Could you check a few things on this model? Use its own coordinates, in mm. A direction names the side the tool comes from. Coordinates: 2 decimals unless noted, no trailing zeros. Order: outer loops, then holes, each group sorted by start corner. A loop starts at its lowest first (then second) coordinate and runs counter-clockwise, first axis right, second up. Notation, with made-up numbers: (-25, -28.5) -> (-2, -28.5) arc R27 cw to (-2, 6.5) -> close; hole circle Ø4 at (9.25, -11.75). An arc over 180 degrees is marked (long way). Put each result on its own line as item: value. Start each with the question number.
Q1. Please list where these lines run through material, in increasing order: line 1 along X through (y, z) = (6, -63); line 2 along X through (y, z) = (5.4, 63.5); line 3 along Z through (x, y) = (111.5, 19.5).
Q2. Will these pins go through, and if not, where does the flat tip stop? pin 1 (19.5 mm diameter, centred on x = 145, y = 20.5, fed in from +Z); pin 2 (11 mm diameter, centred on x = 207.5, z = -66.5, fed in from +Y); pin 3 (4 mm diameter, centred on x = 31.5, z = 49, fed in from +Y).
Q3. For faces 1 (the face through (150, 4.382, 65)), 2 (the face through (150, 38.227, -1)), which set-ups out of +Z, -Z, +X, -X, +Y, -Y let a thin tool reach every point of the face, with its end or its side?
Q4. If we section it at D-D (z = -39): Please give me the cut outline in (x, y) (3 decimals), and give its area (3 significant figures).
Q5. If we section it at A-A (y = 30.5): Please give me the cut outline in (x, z), and give its area (3 significant figures).
Q6. If we section it at C-C (z = 20.5): Please give me the cut outline in (x, y) (3 decimals), and give its area (3 significant figures).
Q7. We'd pull the mould along Z, two halves only. Please class faces 3 (the face through (150.27, 6.25, 49.53)), 4 (the face through (150, 7.43, -65)), 5 (the face through (150, 23, -50.8)): +Z half, -Z half, draft (parallel to the pull), parting line (faces both ways), or undercut.
from build123d import *

# Parameters (mm, degrees)
BOSS_EXTRUDE1_DEPTH              = 304.8
SKETCH2_R                        = 2.3876
CUT_EXTRUDE1_DEPTH               = 317.354227758
SKETCH3_R                        = 9.525
CUT_EXTRUDE2_DEPTH               = 304.8
LPATTERN1_COUNT                  = 2
LPATTERN1_PITCH                  = 171.958
FILLET1_R                        = 6.35
CONVERT_SOLID1_DEPTH             = 304.8
F_10_0_1935_DIAMETER_HOLE1_D     = 4.9149
F_10_0_1935_DIAMETER_HOLE1_DEPTH = 3.048


# Read off the part's stored shape, not the designer's step: Convert-Solid1
with BuildPart() as part:
    # Sketch1 → Boss-Extrude1 (new body)
    with BuildSketch(Plane(origin=(0, 0, 0), x_dir=(0, 0, -1), z_dir=(1, 0, 0))):
        with BuildLine():
            Line((-76.2, 4.2545), (-53.975, 4.2545))
            ThreePointArc((-53.975, 4.2545), (-49.484871939, 6.114371939), (-47.625, 10.6045))
            Line((-47.625, 10.6045), (-47.625, 34.925))
            ThreePointArc((-47.625, 34.925), (-46.69506403, 37.17006403), (-44.45, 38.1))
            Line((-44.45, 38.1), (44.45, 38.1))
            ThreePointArc((44.45, 38.1), (46.69506403, 37.17006403), (47.625, 34.925))
            Line((47.625, 34.925), (47.625, 10.6045))
            ThreePointArc((47.625, 10.6045), (49.484871939, 6.114371939), (53.975, 4.2545))
            Line((53.975, 4.2545), (76.2, 4.2545))
            Line((76.2, 4.2545), (76.2, 7.4295))
            Line((76.2, 7.4295), (53.975, 7.4295))
            ThreePointArc((53.975, 7.4295), (51.72993597, 8.35943597), (50.8, 10.6045))
            Line((50.8, 10.6045), (50.8, 34.925))
            ThreePointArc((50.8, 34.925), (48.940128061, 39.415128061), (44.45, 41.275))
            Line((44.45, 41.275), (-44.45, 41.275))
            ThreePointArc((-44.45, 41.275), (-48.940128061, 39.415128061), (-50.8, 34.925))
            Line((-50.8, 34.925), (-50.8, 10.6045))
            ThreePointArc((-50.8, 10.6045), (-51.72993597, 8.35943597), (-53.975, 7.4295))
            Line((-53.975, 7.4295), (-76.2, 7.4295))
            Line((-76.2, 7.4295), (-76.2, 4.2545))
        make_face()
    extrude(amount=BOSS_EXTRUDE1_DEPTH)

    # Sketch2 → Cut-Extrude1 (cut, through all)
    with BuildSketch(Plane.XZ.offset(-4.2545)):
        with Locations(Location((25.4, 63.5, 0), (0, 0, 270))):
            Circle(SKETCH2_R)
        with Locations(Location((152.4, 63.5, 0), (0, 0, 270))):
            Circle(SKETCH2_R)
        with Locations(Location((279.4, 63.5, 0), (0, 0, 270))):
            Circle(SKETCH2_R)
    cut_extrude1 = extrude(amount=-CUT_EXTRUDE1_DEPTH, mode=Mode.SUBTRACT)

    # Mirror1: Cut-Extrude1 across plane
    add(cut_extrude1.mirror(Plane.XY), mode=Mode.SUBTRACT)

    # Sketch3 → Cut-Extrude2 (cut)
    with BuildSketch(Plane(origin=(0, 41.275, 0), x_dir=(1, 0, 0), z_dir=(0, 1, 0))):
        with Locations(Location((66.675, -15.875, 0), (0, 0, 270))):
            Circle(SKETCH3_R)
    cut_extrude2 = extrude(amount=-CUT_EXTRUDE2_DEPTH, mode=Mode.SUBTRACT)

    # LPattern1: Cut-Extrude2 ×2
    with Locations(*[(i * LPATTERN1_PITCH, 0, 0) for i in range(1, LPATTERN1_COUNT)]):
        add(cut_extrude2, mode=Mode.SUBTRACT)

    # Fillet1
    fillet1_edges = [part.edges().sort_by_distance(p)[0] for p in [
        (0, 5.842, -76.2),
        (0, 5.842, 76.2),
        (304.8, 5.842, -76.2),
        (304.8, 5.842, 76.2),
    ]]
    fillet(fillet1_edges, radius=FILLET1_R)

    # Convert-Solid1 outline → Convert-Solid1 (cut)
    with BuildSketch(Plane.YZ):
        with BuildLine():
            Line((4.3815, -76.2), (4.3815, -53.975))
            ThreePointArc((4.3815, -53.975), (6.204174501, -49.574674501), (10.6045, -47.752))
            Line((10.6045, -47.752), (34.925, -47.752))
            ThreePointArc((34.925, -47.752), (37.259866591, -46.784866591), (38.227, -44.45))
            Line((38.227, -44.45), (38.227, 44.45))
            ThreePointArc((38.227, 44.45), (37.259866591, 46.784866591), (34.925, 47.752))
            Line((34.925, 47.752), (10.6045, 47.752))
            ThreePointArc((10.6045, 47.752), (6.204174501, 49.574674501), (4.3815, 53.975))
            Line((4.3815, 53.975), (4.3815, 76.2))
            Line((4.3815, 76.2), (4.2545, 76.2))
            Line((4.2545, 76.2), (4.2545, 53.975))
            ThreePointArc((4.2545, 53.975), (6.114371939, 49.484871939), (10.6045, 47.625))
            Line((10.6045, 47.625), (34.925, 47.625))
            ThreePointArc((34.925, 47.625), (37.17006403, 46.69506403), (38.1, 44.45))
            Line((38.1, 44.45), (38.1, -44.45))
            ThreePointArc((38.1, -44.45), (37.17006403, -46.69506403), (34.925, -47.625))
            Line((34.925, -47.625), (10.6045, -47.625))
            ThreePointArc((10.6045, -47.625), (6.114371939, -49.484871939), (4.2545, -53.975))
            Line((4.2545, -53.975), (4.2545, -76.2))
            Line((4.2545, -76.2), (4.3815, -76.2))
        make_face()
    extrude(amount=CONVERT_SOLID1_DEPTH, mode=Mode.SUBTRACT)

    # #10 (0.1935) Diameter Hole1
    with Locations(Plane(origin=(0, 7.4295, 0), x_dir=(1, 0, 0), z_dir=(0, 1, 0))):
        with Locations((25.4, 63.5), (152.4, 63.5), (279.4, 63.5), (279.4, -63.5), (152.4, -63.5), (25.4, -63.5)):
            Hole(F_10_0_1935_DIAMETER_HOLE1_D / 2, depth=F_10_0_1935_DIAMETER_HOLE1_DEPTH)


solid = part.part
The answers:
1. line 1: 0 to 22.99, 27.81 to 149.99, 154.81 to 276.99, 281.81 to 304.8
1. line 2: 0 to 22.94, 27.86 to 149.94, 154.86 to 276.94, 281.86 to 304.8
1. line 3: -50.8 to -47.75, 47.75 to 50.8
2. pin 1: z = 50.8
2. pin 2: y = 7.43
2. pin 3: y = 40.74
3. face 1: +Z, -Z, +X, -X, -Y
3. face 2: +X, -X, -Y
4. outline: (0, 38.227) -> (304.8, 38.227) -> (304.8, 41.275) -> (0, 41.275) -> close
4. area: 929 mm^2
5. outline: (0, -50.8) -> (304.8, -50.8) -> (304.8, -47.75) -> (0, -47.75) -> close; (0, 47.75) -> (304.8, 47.75) -> (304.8, 50.8) -> (0, 50.8) -> close
5. area: 1,860 mm^2
6. outline: (0, 38.227) -> (58.348, 38.227) -> (58.348, 41.275) -> (0, 41.275) -> close; (75.002, 38.227) -> (230.306, 38.227) -> (230.306, 41.275) -> (75.002, 41.275) -> close; (246.96, 38.227) -> (304.8, 38.227) -> (304.8, 41.275) -> (246.96, 41.275) -> close
6. area: 828 mm^2
7. face 3: undercut
7. face 4: draft
7. face 5: -Z half
